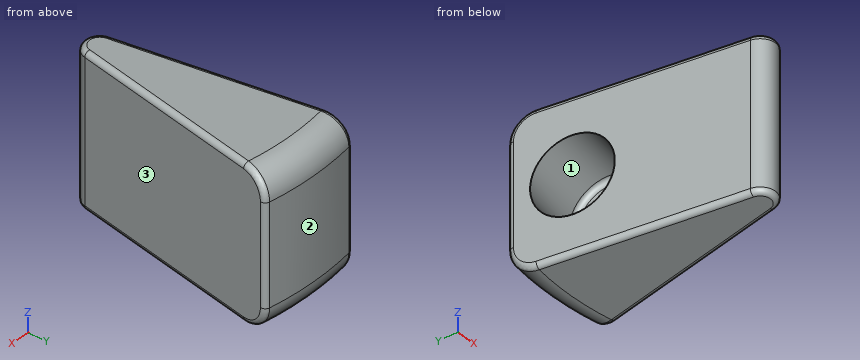
```python
from build123d import *

# Parameters (mm, degrees)
F1_ANGLE_BACK = 10
F1_ANGLE      = 20
F2_R          = 3
F3_R          = 7.5
F4_DEPTH      = 13
F5_R          = 1


with BuildPart() as f1:
    # F0 (on Right) → F1 (revolve)
    with BuildSketch(Plane.YZ, mode=Mode.PRIVATE) as f1_sk:
        with BuildLine():
            ThreePointArc((30, 10), (28.5355339059, 13.5355339059), (25, 15))
            Line((25, 15), (-30, 15))
            Line((-30, 15), (-30, -15))
            Line((-30, -15), (25, -15))
            ThreePointArc((25, -15), (28.5355339059, -13.5355339059), (30, -10))
            Line((30, -10), (30, 10))
        make_face()
    revolve(f1_sk.sketch.rotate(Axis((0, -30, 0), (0, 0, -1)), -F1_ANGLE_BACK), axis=Axis((0, -30, 0), (0, 0, -1)), revolution_arc=F1_ANGLE)

    # F2
    f2_edges = [f1.edges().sort_by_distance(p)[0] for p in [
        (0, -30, 0),
    ]]
    fillet(f2_edges, radius=F2_R)

    # F3 (on face) → F4 (cut)
    with BuildSketch(Plane(origin=(-5.1303021499, -0.9046106882, 0), x_dir=(0.1736481777, -0.984807753, 0), z_dir=(-0.984807753, -0.1736481777, 0))):
        with Locations((-19, 0)):
            Circle(F3_R)
    extrude(amount=-F4_DEPTH, mode=Mode.SUBTRACT)

    # F5
    f5_edges = [f1.edges().sort_by_distance(p)[0] for p in [
        (10.164589, 27.646248, -13.535534),
        (3.070522, 27.450221, 0),
    ]]
    fillet(f5_edges, radius=F5_R)


solid = f1.part
```
For this review, take the finished solid that the model builds, in its own axes (mm). Face numbers are marked on the shaded views. Coordinates: 2 decimals unless noted, no trailing zeros. Loops run counter-clockwise (first coordinate to the right, second up) from the corner with the lowest first, then second, coordinate; pieces in that order, holes last.
1. Add section A-A, the plane z = 8.5. Give the boundary of the cut face in (x, y).
2. Mouldability with a two-part tool opening along Y and no side actions: class the marked faces 1, 2 and 3 as +Y half, -Y half, draft (parallel to the pull), parting line (faces both ways), or undercut.
3. For line 1 (Z direction, x = -8, y = 20.5); line 2 (Z direction, x = -2.5, y = 23); line 3 (X direction, y = -5, z = 4.5), list the stretches that pass through material, from the lowest coordinate up.
4. Insertion check: P1, Ø12, axis at y = -5, z = 9.5, coming from the +X side; P2, Ø4, axis at y = 18, z = -6.5, coming from the +X side; P3, Ø3, axis at y = 8, z = 10.5, coming from the +X side. Each pin has a flat end and moves straight along its axis. Give the tip position at first contact, or say it passes through.
Result:
1. outline: (-10.24, 28.1) - (-2.95, -13.24) arc R3 ccw to (2.95, -13.24) - (10.24, 28.1) arc R1 ccw to (9.42, 29.26) arc R60 ccw to (-9.42, 29.26) arc R1 ccw to start
2. face 1: undercut
2. face 2: +Y half
2. face 3: -Y half
3. line 1: z = -14.99 to -7.04, 7.04 to 14.99
3. line 2: z = -15 to -6.29, 6.29 to 15
3. line 3: x = -4.41 to 4.41
4. P1: stops at x = 5.47
4. P2: stops at x = 8.82
4. P3: stops at x = 6.96
